Autodesk Inventor part; units mm, degrees
ref_plane "YZ Plane" through (0, 0, 0) normal (1, 0, 0) x (0, 1, 0)
ref_plane "XZ Plane" through (0, 0, 0) normal (0, 1, 0) x (-1, 0, 0)
ref_plane "XY Plane" through (0, 0, 0) normal (0, 0, 1) x (1, 0, 0)
sketch "Boceto1" plane through (0, 0, 0) normal (0, 0, 1) x (1, 0, 0)
  line L0 (49.5506, 21.8243) -> (55.5506, 21.8243)
  line L1 (55.5506, 21.8243) -> (55.5506, -21.1757)
  line L2 (55.5506, -21.1757) -> (12.5506, -21.1757)
  line L3 (12.5506, -21.1757) -> (12.5506, -15.1757)
  line L4 (55.5506, 21.8243) -> (49.5506, 21.8243)
  line L5 (12.5506, -21.1757) -> (12.5506, -15.1757)
  line L6 (12.5506, -15.1757) -> (49.5506, 21.8243)
  circle A0 centre (40.1551, -5.7801) radius 3
  point P0 (0, 0)
  dimension "d0" = 43
  dimension "d1" = 43
  dimension "d2" = 6
  dimension "d3" = 6
  dimension "d4" = 6
extrude "Extrusión1" add sketch "Boceto1" along normal blind 3
sketch "Boceto2" plane through (0, 0, 3) normal (0, 0, 1) x (1, 0, 0)
  line L0 (12.5506, -15.1757) -> (12.5506, -21.1757)
  line L1 (55.5506, -21.1757) -> (55.5506, 21.8243)
  line L2 (12.5506, -21.1757) -> (55.5506, -21.1757)
  line L3 (55.5506, -21.1757) -> (55.5506, -18.1757)
  line L4 (55.5506, -18.1757) -> (12.5506, -18.1757)
  line L5 (12.5506, -18.1757) -> (12.5506, -21.1757)
  point P0 (0, 0)
  dimension "d7" = 3
extrude "Extrusión2" add sketch "Boceto2" along normal blind 27
sketch "Boceto3" plane through (0, 0, 3) normal (0, 0, 1) x (1, 0, 0)
  line L0 (12.5506, -18.1757) -> (55.5506, -18.1757)
  line L1 (55.5506, 21.8243) -> (49.5506, 21.8243)
  line L2 (55.5506, -18.1757) -> (52.5506, -18.1757)
  line L3 (52.5506, -18.1757) -> (52.5506, 21.8243)
  line L4 (52.5506, 21.8243) -> (55.5506, 21.8243)
  line L5 (55.5506, 21.8243) -> (55.5506, -18.1757)
  point P0 (0, 0)
extrude "Extrusión3" add sketch "Boceto3" along normal blind 27
fillet "Empalme1" radius 2 1 edges at (34.0506, -21.1757, 0)
sketch "Boceto4" plane through (52.5506, -18.1757, 3) normal (-1, 0, 0) x (0, 0, 1)
  line L0 (-3, 40) -> (27, 40)
  line L1 (27, 40) -> (12, 40)
  line L2 (-1, -3) -> (27, -3)
  line L3 (16.5, 26) -> (16.5, 13)
  line L4 (7.5, 13) -> (7.5, 26)
  line L5 (27, 40) -> (27, 0)
  arc A0 (16.5, 26) -> (7.5, 26) centre (12, 26) ccw
  arc A1 (7.5, 13) -> (16.5, 13) centre (12, 13) ccw
  point P0 (-3, 18.1757)
  dimension "d13" = 15
  dimension "d15" = 9
  dimension "d16" = 13
  dimension "d19" = 9
  dimension "d20" = 9
extrude "Extrusión4" cut sketch "Boceto4" against normal blind 3
sketch "Boceto5" plane through (12.5506, -18.1757, 30) normal (0, 1, 0) x (1, 0, 0)
  line L0 (0, 30) -> (0, 15)
  line L1 (0, 28) -> (0, 0)
  line L2 (43, 19.5) -> (43, 10.5)
  line L3 (15, 10.5) -> (28, 10.5)
  line L4 (28, 19.5) -> (15, 19.5)
  line L5 (37, 30) -> (0, 30)
  arc A0 (15, 19.5) -> (15, 10.5) centre (15, 15) ccw
  arc A1 (28, 10.5) -> (28, 19.5) centre (28, 15) ccw
  point P0 (-12.5506, 30)
  dimension "d23" = 15
  dimension "d28" = 19.5
extrude "Extrusión5" cut sketch "Boceto5" against normal blind 3
sketch "Boceto6" plane through (52.5506, -18.1757, 3) normal (-1, 0, 0) x (0, 0, 1)
  point P0 (-3, 18.1757)
properties part number "Sujetador2" material "Acero, galvanizado"
For this review, take the finished solid that the model builds, in its own axes (mm). A direction names the side the tool comes from. Give positions to 0.01 mm unless a question says otherwise; leave off trailing zeros. Loops run counter-clockwise (first coordinate to the right, second up) from the corner with the lowest first, then second, coordinate; pieces in that order, holes last. Notation, with made-up numbers: M 26.25,-13.75 L 37.25,-13.75 A13 ccw 37.25,10.25 Z; hole C -5.5,30.5 d10. An arc over 180 degrees is marked long. Answer as a JSON object with one key per item and string values. Group by question number.
Q1. Insertion check: P1, Ø5, axis at x = 20.5, z = 13, coming from the +Y side; P2, Ø8, axis at y = -2.5, z = 11, coming from the -X side. Each pin has a flat end and moves straight along its axis. Give the tip position at first contact, or say it passes through.
Q2. Add section B-B on y = 4.5. Give the boundary of the cut face in (x, z), and give its area (3 significant figures).
Q3. Add section D-D on x = 26.5. Give the boundary of the cut face in (y, z).
Q4. Add section A-A on z = 15. Give the boundary of the cut face in (x, y).
Q5. Mouldability with a two-part tool opening along Y and no side actions: class faces 1 (the cylindrical face through (33.75, -20.574, 0.57)), 2 (the cylindrical face through (23.05, -19.65, 14.9)), 3 (the flat face through (54, 1, 10.5)) as +Y half, -Y half, draft (parallel to the pull), parting line (faces both ways), or undercut.
Q6. For probe 1 along X at (y, z) = (-14.5, 22); probe 2 along Z at (x, y) = (33, -11); probe 3 along Y at (x, z) = (17, 14.5), list the stretches that pass through material, from the lowest coordinate up. Write a range as [from, to].
Q7. Add section C-C on x = 22. Give the boundary of the cut face in (y, z).
Q8. Tool access review of faces 4 (the cylindrical face through (42.926, -4.631, 1.479)), 5 (the flat face through (12.551, -20, 15)), 6 (the flat face through (54, 1, 19.5)), 7 (the flat face through (34, -20, 10.5)), 8 (the flat face through (33, -18.176, 22)): name each direction out of +Z, -Z, +X, -X, +Y, -Y from which nothing blocks a thin tool from reaching the whole face with its end or side.
Checked values:
{
 "1": {"P1": "y = -18.18", "P2": "x = 52.55"},
 "2": {"outline": "M 32.23,0 L 55.55,0 L 55.55,10.5 L 52.55,10.5 L 52.55,3 L 32.23,3 Z; M 52.55,19.5 L 55.55,19.5 L 55.55,30 L 52.55,30 Z", "area": "124 mm²"},
 "3": {"outline": "M -21.18,2 A2 ccw -19.18,0 L -1.23,0 L -1.23,3 L -18.18,3 L -18.18,10.62 L -21.18,10.62 Z; M -21.18,19.38 L -18.18,19.38 L -18.18,30 L -21.18,30 Z"},
 "4": {"outline": "M 12.55,-21.18 L 23.05,-21.18 L 23.05,-18.18 L 12.55,-18.18 Z; M 45.05,-21.18 L 55.55,-21.18 L 55.55,-9.68 L 52.55,-9.68 L 52.55,-18.18 L 45.05,-18.18 Z; M 52.55,12.32 L 55.55,12.32 L 55.55,21.82 L 52.55,21.82 Z"},
 "5": {"face 1": "-Y half", "face 2": "draft", "face 3": "undercut"},
 "6": {"probe 1": "[52.55, 55.55]", "probe 2": "[0, 3]", "probe 3": "[-21.18, -18.18]"},
 "7": {"outline": "M -21.18,2 A2 ccw -19.18,0 L -5.73,0 L -5.73,3 L -18.18,3 L -18.18,30 L -21.18,30 Z"},
 "8": {"face 4": "+Z, -Z", "face 5": "+Z, -Z, -X, +Y, -Y", "face 6": "+X, -X", "face 7": "+Y, -Y", "face 8": "+Z, -X, +Y"}
}
